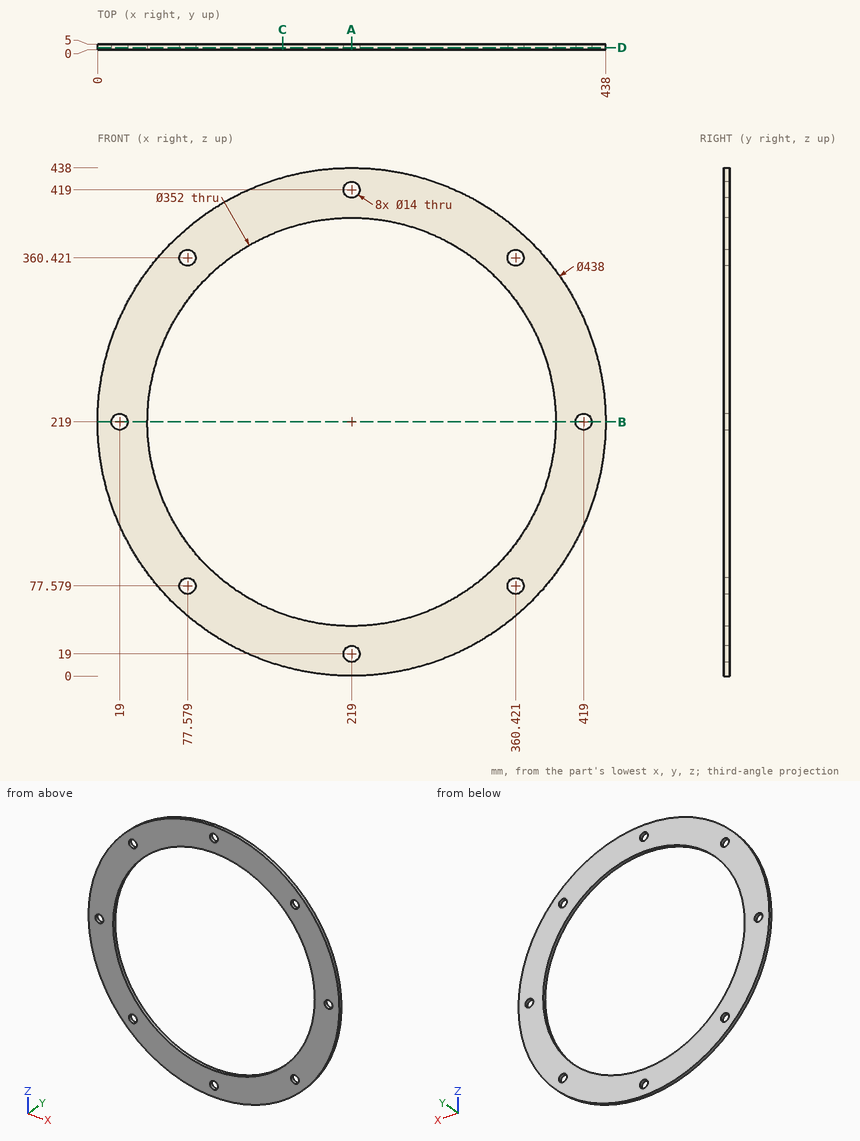
Can you work these out from the drawing? Everything is in mm from the part's minimum corner. Round coordinates to 2 decimals unless told otherwise and drop trailing zeros. Loops run counter-clockwise (first coordinate to the right, second up) from the corner with the lowest first, then second, coordinate; pieces in that order, holes last. Notation, with made-up numbers: (75, 1) - (116, 1) arc R19 cw to (116, 37) - close; hole circle Ø3 at (81.25, -8). An arc over 180 degrees is marked (long way). One line per question, with ' | ' between items. Start each with the question number.
Q1. I want a section at C-C (x = 159.5). Write out the boundary of the cut face in (y, z).
Q2. Please list where these lines run through material, in increasing order: line 1 (X direction, y = 2.15, z = 219); line 2 (X direction, y = 4.25, z = 115) (1 decimal); line 3 (Z direction, x = 307.5, y = 2). Write a range as [from, to].
Q3. I want a section at B-B (z = 219). Write out the boundary of the cut face in (x, y), then the cut area to 3 significant figures.
Q4. Will this pin go through, and if not, where does the flat tip stop? pin 1 (1.5 mm diameter, centred on y = 4.5, z = 139, fed in from -X).
Q5. I want a section at D-D (y = 1.8). State how many separate pieces and enclosed holes the cut face has, then the cut area to 3 significant figures.
Q6. I want a section at A-A (x = 219). Write out the boundary of the cut face in (y, z).
Response values:
1) outline: (0, 8.24) - (5, 8.24) - (5, 53.36) - (0, 53.36) - close; (0, 384.64) - (5, 384.64) - (5, 429.76) - (0, 429.76) - close
2) line 1: x = [0, 12], [26, 43], [395, 412], [426, 438] | line 2: x = [26.3, 77], [361, 411.7] | line 3: z = [18.68, 66.87], [371.13, 419.32]
3) outline: (0, 0) - (12, 0) - (12, 5) - (0, 5) - close; (26, 0) - (43, 0) - (43, 5) - (26, 5) - close; (395, 0) - (412, 0) - (412, 5) - (395, 5) - close; (426, 0) - (438, 0) - (438, 5) - (426, 5) - close | area: 290 mm²
4) pin 1: stops at x = 14.84
5) separate pieces: 1 | enclosed holes: 9 | area: 52,100 mm²
6) outline: (0, 0) - (5, 0) - (5, 12) - (0, 12) - close; (0, 26) - (5, 26) - (5, 43) - (0, 43) - close; (0, 395) - (5, 395) - (5, 412) - (0, 412) - close; (0, 426) - (5, 426) - (5, 438) - (0, 438) - close
